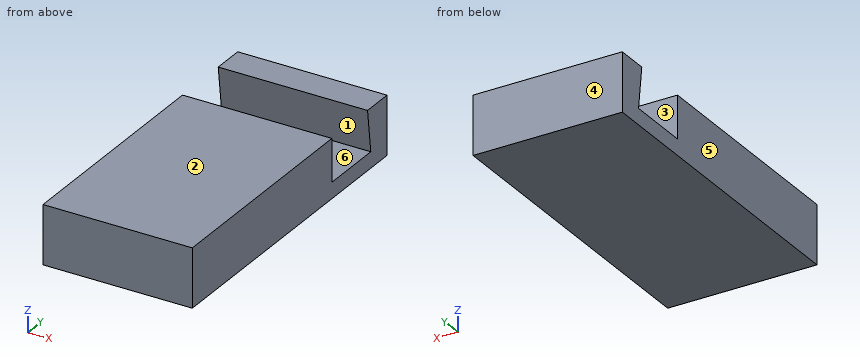
```python
from build123d import *

# Parameters (mm, degrees)
PAD_DEPTH = 14


with BuildPart() as part:
    # Sketch → Pad (new body, symmetric)
    with BuildSketch(Plane.YZ):
        Polygon((0, 11), (0, 0), (60, 0), (60, 11), (54, 11), (55, 3), (43, 3), (43, 11), align=None)
    extrude(amount=PAD_DEPTH, both=True)


solid = part.part
```
Geometry check sheet. Reference: the model listing, model coordinates, mm. Face numbers are marked on the shaded views. A direction names the side the tool comes from. Round coordinates to 2 decimals unless told otherwise and drop trailing zeros. Loops run counter-clockwise (first coordinate to the right, second up) from the corner with the lowest first, then second, coordinate; pieces in that order, holes last. Notation, with made-up numbers: (75, 32) - (117, 32) arc R21 ccw to (117, 66) - close; hole circle Ø3 at (83.5, 26). An arc over 180 degrees is marked (long way). Write each question's results on one line, items separated by ' | '. Start each with the question number.
Q1. Cross-section at B-B on x = -5.5. Enter the section's corners in (y, z), and give its area (3 significant figures).
Q2. Cross-section at A-A on z = 7. Enter the section's corners in (x, y).
Q3. Cross-section at C-C on z = 9.75. Enter the section's corners in (x, y), and give its area (3 significant figures).
Q4. Access from +Z, -Z, +X, -X, +Y, -Y to the whole of each face (thin tool, end or side, straight path). Record for the marked faces 1, 2 and 3.
Q5. Cross-section at D-D on y = 49.5. Enter the section's corners in (x, z).
Q6. Thickness scan on line 1 (Z direction, x = -2.25, y = 45.5); line 2 (Y direction, x = 2, z = 10.75); line 3 (Y direction, x = 1.75, z = 8.25). Record the ranges inside material, lowest first. Write a range as [from, to].
Q7. Release check for a two-part mould opening along Y. For the marked faces 4, 5 and 6 record: +Y half, -Y half, draft (parallel to the pull), parting line (faces both ways), or undercut.
Answers below:
1) outline: (0, 0) - (60, 0) - (60, 11) - (54, 11) - (55, 3) - (43, 3) - (43, 11) - (0, 11) - close | area: 568 mm²
2) outline: (-14, 0) - (14, 0) - (14, 43) - (-14, 43) - close; (-14, 54.5) - (14, 54.5) - (14, 60) - (-14, 60) - close
3) outline: (-14, 0) - (14, 0) - (14, 43) - (-14, 43) - close; (-14, 54.16) - (14, 54.16) - (14, 60) - (-14, 60) - close | area: 1,370 mm²
4) face 1: +X, -X | face 2: +Z, +X, -X, +Y, -Y | face 3: +Z, +X, -X
5) outline: (-14, 0) - (14, 0) - (14, 3) - (-14, 3) - close
6) line 1: z = [0, 3] | line 2: y = [0, 43], [54.03, 60] | line 3: y = [0, 43], [54.34, 60]
7) face 4: +Y half | face 5: draft | face 6: undercut
